The listing builds one solid part. Answer for the finished solid, in the listing's coordinates (mm). A direction names the side the tool comes from. Round coordinates to 2 decimals unless told otherwise and drop trailing zeros. Write each loop counter-clockwise with the first axis right and the second up, starting at its lowest first coordinate (ties: lowest second). Pieces come first, ordered by that corner, then holes.
(1) A cutting plane is placed at A-A, the plane z = 1.45. Give the number of separate pieces and of enclosed holes in the cut face, and give its area (3 significant figures).
(2) Each of these flat-tipped pins is pushed along its axis until it touches: pin 1 Ø0.6 at (y, z) = (13, 1) entering from -X; pin 2 Ø0.6 at (x, z) = (9.5, 1) entering from -Y. Where does it stop, or does it pass through?
(3) A cutting plane is placed at C-C, the plane y = -4. Give the vertices of the cut face in (x, z), and give its area (3 significant figures).
(4) For faces 1 (the face through (14, 40.571, 1)), 2 (the face through (-44.644, 53.91, 1.064)), 3 (the face through (-29.915, 9, 1)), determine the directions among +Z, -Z, +X, -X, +Y, -Y from which every point of the face is accessible in a straight line to the end or side of a thin tool.
(5) The mould has two halves that part along X. Classify faces 4 (the face through (-49, 40.571, 1)), 5 (the face through (-19.18, 39.76, 1.06)), 6 (the face through (-60.601, 41.665, 1.064)), 7 (the face through (-18.359, 29.665, 1.064)): +X half, -X half, draft (parallel to the pull), parting line (faces both ways), or undercut.
(6) Find the intervals of material crossed by probe 1 along X at (y, z) = (-10.5, 0.4); probe 2 along X at (y, z) = (-1.5, 1.7); probe 3 along Y at (x, z) = (16, 0.85), in increasing order.
(7) A cutting plane is placed at B-B, the plane x = 15.5. Give the vertices of the cut face in (y, z).
from build123d import *

# Parameters (mm, degrees)
SKETCH1_W                   = 25.4
SKETCH1_H                   = 57.15
BOSS_EXTRUDE1_DEPTH         = 2.159
FILLET1_R                   = 7.62
CHAMFER1_SIZE               = 2.159
F_1_4_0_25_DIAMETER_HOLE1_D = 4.2545


with BuildPart() as part:
    # Sketch1 → Boss-Extrude1 (new body)
    with BuildSketch(Plane.XY):
        Polygon((27.234954785, 40.570800108), (-4.515045215, 40.570800108), (-29.915045215, 40.570800108), (-61.665045215, 40.570800108), (-61.665045215, 65.970800108), (27.234954785, 65.970800108), align=None)
        with Locations((-17.215045215, 11.995800108)):
            Rectangle(SKETCH1_W, SKETCH1_H)
    extrude(amount=BOSS_EXTRUDE1_DEPTH)

    # Fillet1
    fillet1_edges = [part.edges().sort_by_distance(p)[0] for p in [
        (-4.515045215, 40.570800108, 1.0795),
        (-29.915045215, 40.570800108, 1.0795),
    ]]
    fillet(fillet1_edges, radius=FILLET1_R)

    # Chamfer1
    chamfer1_edges = [part.edges().sort_by_distance(p)[0] for p in [
        (-4.515045215, -16.579199892, 1.0795),
        (-29.915045215, -16.579199892, 1.0795),
        (-61.665045215, 40.570800108, 1.0795),
        (-61.665045215, 65.970800108, 1.0795),
        (27.234954785, 65.970800108, 1.0795),
        (27.234954785, 40.570800108, 1.0795),
    ]]
    chamfer(chamfer1_edges, length=CHAMFER1_SIZE)

    # 1/4 (0.25) Diameter Hole1 (through all)
    with Locations(Plane.XY.offset(2.159)):
        with Locations((-55.315045215, 53.270800108), (-42.615045215, 53.270800108), (-29.915045215, 53.270800108), (-17.215045215, 53.270800108), (-4.515045215, 53.270800108), (8.184954785, 53.270800108), (20.884954785, 53.270800108), (-17.215045215, 40.570800108), (-17.215045215, 27.870800108), (-17.215045215, 15.170800108), (-17.215045215, 2.470800108), (-17.215045215, -10.229199892)):
            Hole(F_1_4_0_25_DIAMETER_HOLE1_D / 2)


solid = part.part
Solutions:
1. separate pieces: 1
1. enclosed holes: 12
1. area: 3,550 mm2
2. pin 1: stops at x = -29.92
2. pin 2: stops at y = 40.57
3. outline: (-29.92, 0) - (-4.52, 0) - (-4.52, 2.16) - (-29.92, 2.16) - close
3. area: 54.8 mm2
4. face 1: +Z, -Z, +X, -Y
4. face 2: +Z, -Z
4. face 3: +Z, -Z, -X, -Y
5. face 4: draft
5. face 5: undercut
5. face 6: -X half
5. face 7: undercut
6. probe 1: x = -29.92 to -19.32, -15.11 to -4.52
6. probe 2: x = -29.92 to -4.52
6. probe 3: y = 40.57 to 65.97
7. outline: (40.57, 0) - (65.97, 0) - (65.97, 2.16) - (40.57, 2.16) - close
